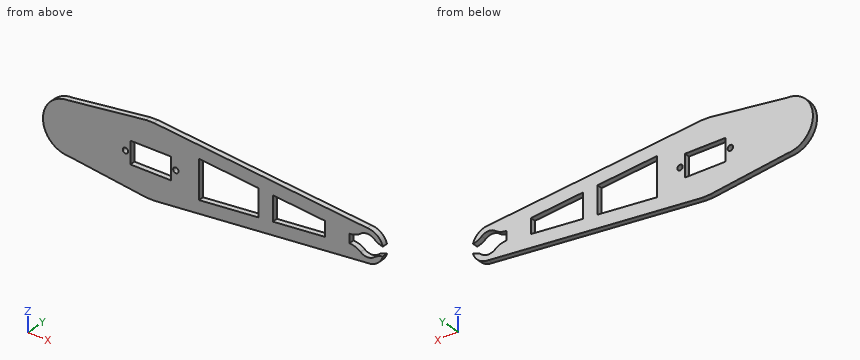
```python
from build123d import *

# Parameters (mm, degrees)
SKETCH1_R           = 1.5
SKETCH1_R_2         = 6
SKETCH1_W           = 22.5
SKETCH1_H           = 12.2
BOSS_EXTRUDE1_DEPTH = 3
SKETCH3_W           = 20
SKETCH3_H           = 5
CUT_EXTRUDE1_DEPTH  = 131.520857309
FILLET1_R           = 10


with BuildPart() as part:
    # Sketch1 → Boss-Extrude1 (new body)
    with BuildSketch(Plane(origin=(0, 0, 0), x_dir=(1, 0, 0), z_dir=(0, 1, 0))):
        with BuildLine():
            Line((1.846751087, 19.91455524), (120, 8.957763171))
            ThreePointArc((120, 8.957763171), (128.957763171, 0), (120, -8.957763171))
            Line((120, -8.957763171), (1.846751087, -19.91455524))
            Line((1.846751087, -19.91455524), (-2.565887989, -19.834722555))
            Line((-2.565887989, -19.834722555), (-45.343490518, -14.300864634))
            ThreePointArc((-45.343490518, -14.300864634), (-59.644355152, 0), (-45.343490518, 14.300864634))
            Line((-45.343490518, 14.300864634), (-2.565887989, 19.834722555))
            Line((-2.565887989, 19.834722555), (1.846751087, 19.91455524))
        make_face()
        with Locations(Location((13.95, 0, 0), (0, 0, 270))):
            Circle(SKETCH1_R, mode=Mode.SUBTRACT)
        with Locations(Location((-13.95, 0, 0), (0, 0, 270))):
            Circle(SKETCH1_R, mode=Mode.SUBTRACT)
        with Locations(Location((120, 0, 0), (0, 0, 270))):
            Circle(SKETCH1_R_2, mode=Mode.SUBTRACT)
        Rectangle(SKETCH1_W, SKETCH1_H, mode=Mode.SUBTRACT)
        Polygon((96.529167285, 4.104267173), (67.660347399, 6.781380665), (67.660347399, -6.781380665), (96.529167285, -4.104267173), align=None, mode=Mode.SUBTRACT)
        Polygon((59.65913304, 7.523363157), (26.779600723, 10.572404992), (26.779600723, -10.572404992), (59.65913304, -7.523363157), align=None, mode=Mode.SUBTRACT)
    extrude(amount=BOSS_EXTRUDE1_DEPTH)

    # Sketch3 → Cut-Extrude1 (cut, through all)
    with BuildSketch(Plane(origin=(0, 3, 0), x_dir=(1, 0, 0), z_dir=(0, 1, 0))):
        with Locations((120, 0)):
            Rectangle(SKETCH3_W, SKETCH3_H)
    extrude(amount=-CUT_EXTRUDE1_DEPTH, mode=Mode.SUBTRACT)

    # Fillet1
    # the kernel refuses this fillet: 10 mm, written as the material it takes off along each edge
    with BuildSketch(Plane(origin=(125.454356057, 10.868690914, 2.5), x_dir=(1, 0, 0), z_dir=(0, -1, 0))) as fillet1_piece_1:
        with BuildLine():
            CenterArc((4.679032278, 9.882020871), FILLET1_R, 230.703265247, 30.48689252)
            Line((-1.654335431, 2.143257826), (-1.781002786, 1.988482566))
            ThreePointArc((-1.781002786, 1.988482566), (-0.863019038, 1.043956035), (-0.181811869, -0.083333333))
            Line((-0.181811869, -0.083333333), (0, -0.2))
            ThreePointArc((0, -0.2), (1.573738183, -0.2), (3.116845247, -0.197640417))
            Line((3.116845247, -0.197640417), (3.147476366, 0))
        make_face()
    extrude(amount=18.737381828, mode=Mode.SUBTRACT)
    with BuildSketch(Plane(origin=(114.545643943, 14.332840301, 2.5), x_dir=(0.6156579371182371, 0, 0.7880135179445317), z_dir=(0, -1, 0))) as fillet1_piece_2:
        with BuildLine():
            CenterArc((5.089273947, 9.728751913), FILLET1_R, 217.99974274, 38.624832873)
            Line((-2.790861233, 3.572172542), (-2.948463936, 3.449040954))
            Line((-2.948463936, 3.449040954), (-0.157602704, -0.123131587))
            Line((-0.157602704, -0.123131587), (0.046266127, -0.194575038))
            ThreePointArc((0.046266127, -0.194575038), (1.387983804, -0.037251148), (2.729701481, -0.194575038))
            Line((2.729701481, -0.194575038), (2.775967607, 0))
        make_face()
    extrude(amount=25.665680602, mode=Mode.SUBTRACT)
    with BuildSketch(Plane(origin=(114.545643943, 14.332840301, -2.5), x_dir=(-1, 0, 0), z_dir=(0, -1, 0))) as fillet1_piece_3:
        with BuildLine():
            CenterArc((4.53313612, 10), FILLET1_R, 231.375167127, 38.624832873)
            Line((-1.709046491, 2.1875), (-1.833890143, 2.03125))
            ThreePointArc((-1.833890143, 2.03125), (-0.883877653, 1.070816035), (-0.181811869, -0.083333333))
            Line((-0.181811869, -0.083333333), (0, -0.2))
            Line((0, -0.2), (4.53313612, -0.2))
            Line((4.53313612, -0.2), (4.53313612, 0))
        make_face()
    extrude(amount=25.665680602, mode=Mode.SUBTRACT)
    with BuildSketch(Plane(origin=(125.454356057, 10.868690914, -2.5), x_dir=(-0.6110269025667731, 0, -0.7916098308760795), z_dir=(0, -1, 0))) as fillet1_piece_4:
        with BuildLine():
            CenterArc((4.96369027, 9.742148554), FILLET1_R, 226.473634032, 30.48689252)
            Line((-1.923192735, 2.491573233), (-2.060930395, 2.346561727))
            ThreePointArc((-2.060930395, 2.346561727), (-1.119918333, 1.123581236), (-0.158321966, -0.122205381))
            Line((-0.158321966, -0.122205381), (0.045124457, -0.194842971))
            ThreePointArc((0.045124457, -0.194842971), (1.35373371, -0.045289132), (2.662342963, -0.194842971))
            Line((2.662342963, -0.194842971), (2.70746742, 0))
        make_face()
    extrude(amount=18.737381828, mode=Mode.SUBTRACT)


solid = part.part
```
Geometry: final body of the model. Coordinates: model frame, mm. Round coordinates to 2 decimals unless told otherwise and drop trailing zeros. Order: outer loops, then holes, each group sorted by start corner. A loop starts at its lowest first (then second) coordinate and runs counter-clockwise, first axis right, second up. Notation, with made-up numbers: (-17.5, 29.25) - (37.5, 29.25) arc R29 ccw to (37.5, 55.25) - close; hole circle Ø2 at (-18.5, 40). An arc over 180 degrees is marked (long way). Use CSV: the item, a comma, the result in double quotes. Start each with the question number.
Q1. Section query A-A (y = 1.8). State how many separate pieces and enclosed holes the cut face has, and give its area (3 significant figures).
Q2. Section query B-B (x = 75.5). Return loops of the section in (y, z).
Q3. First-contact query: pin 1 (0.9 mm diameter, centred on x = -4.5, y = 2, fed in from +Z); pin 2 (0.9 mm diameter, centred on y = 2, z = 1, fed in from -X). Flat tips, straight axial feed; report the tip coordinate or a pass-through.
Q4. Material intervals for line 1 along X through (y, z) = (0.7, 0); line 2 along Z through (x, y) = (-2.5, 1.2); line 3 along Z through (x, y) = (39, 2.65), sorted ascending. Write a range as from..to.
Result set:
1,separate pieces,"1"
1,enclosed holes,"5"
1,area,"4,140 mm2"
2,outline,"(0, -13.08) - (3, -13.08) - (3, -6.05) - (0, -6.05) - close; (0, 6.05) - (3, 6.05) - (3, 13.08) - (0, 13.08) - close"
3,pin 1,"stops at z = 19.64"
3,pin 2,"stops at x = -59.63"
4,line 1,"x = -59.64..-15.45, -12.45..-11.25, 11.25..12.45, 15.45..26.78, 59.66..67.66, 96.53..110"
4,line 2,"z = -19.84..-6.1, 6.1..19.84"
4,line 3,"z = -16.47..-9.44, 9.44..16.47"
